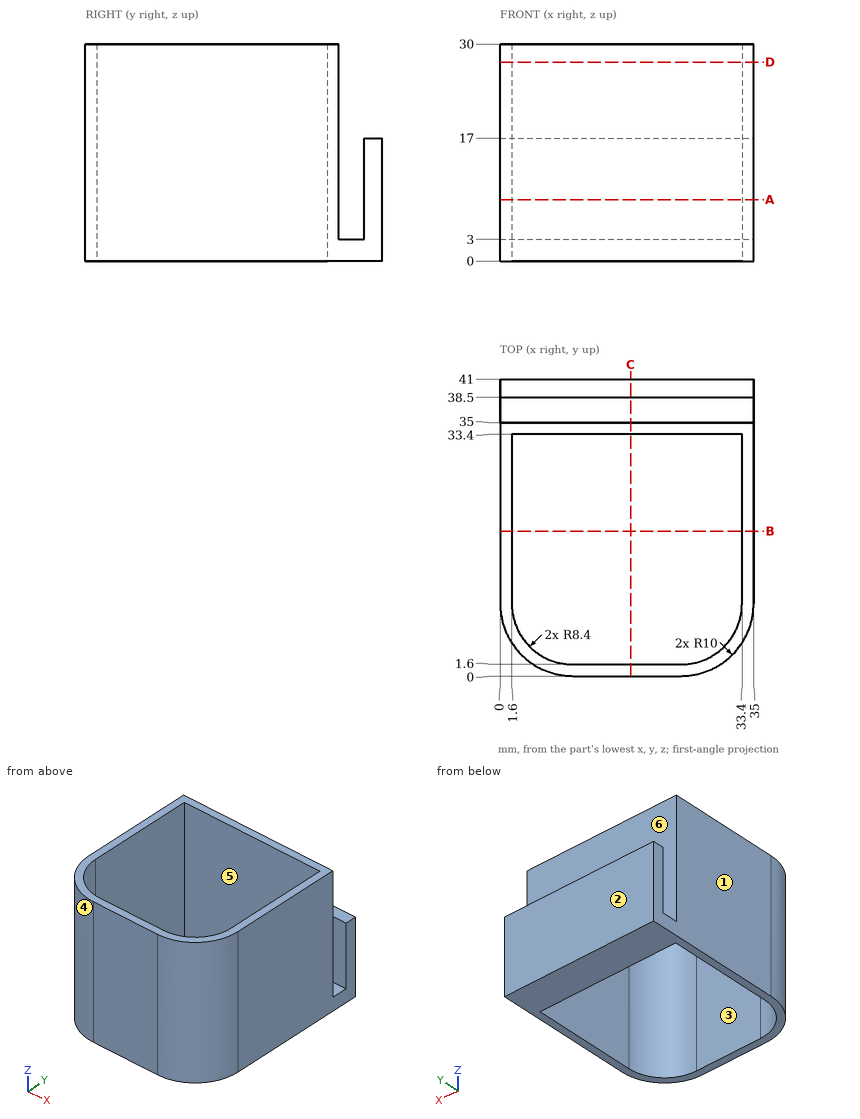
Verification items for this drawing (mm, ordinates from the low corner). A direction names the side the tool comes from. Coordinates: 2 decimals unless noted, no trailing zeros. Order: outer loops, then holes, each group sorted by start corner. A loop starts at its lowest first (then second) coordinate and runs counter-clockwise, first axis right, second up. Notation, with made-up numbers: (31, 56) - (46, 56) arc R12 cw to (46, 64) - close; hole circle Ø3 at (-24, 19). An arc over 180 degrees is marked (long way). Answer as a JSON object with one key per item and string values. Group by question number.
Item 1: Depth check by flat-ended pin: pin 1 Ø1.2 at (x, y) = (15, 40) entering from +Z; pin 2 Ø10 at (x, y) = (11.5, 11.5) entering from +Z. Enter the tip coordinate at first touch or a pass-through.
Item 2: Draft check along X on the marked faces 1, 2 and 3. Enter one of: +X half, -X half, draft (parallel to the pull), parting line (faces both ways), or undercut.
Item 3: Sectioned sample at A-A, the plane z = 8.5. Record the cut outline in (x, y), and give its area (3 significant figures).
Item 4: Sectioned sample at B-B, the plane y = 20. Record the cut outline in (x, z), and give its area (3 significant figures).
Item 5: Scan lines: probe 1 along Y at (x, z) = (23, 8.5); probe 2 along X at (y, z) = (27.5, 1.75); probe 3 along Y at (x, z) = (28, 10.25). Record each from-to range of solid material in increasing order.
Item 6: Tool access check on the marked faces 4, 5 and 6. Record the directions out of +Z, -Z, +X, -X, +Y, -Y that give a thin tool (end or side, any length) a straight path to the whole face; none if there is none.
Item 7: Sectioned sample at D-D, the plane z = 27.5. Record the cut outline in (x, y), and give its area (3 significant figures).
Item 8: Sectioned sample at C-C, the plane x = 18. Record the cut outline in (y, z).
Resolved:
{
 "1": {"pin 1": "z = 17", "pin 2": "through"},
 "2": {"face 1": "-X half", "face 2": "draft", "face 3": "undercut"},
 "3": {"outline": "(0, 10) arc R10 ccw to (10, 0) - (25, 0) arc R10 ccw to (35, 10) - (35, 35) - (0, 35) - close; (0, 38.5) - (35, 38.5) - (35, 41) - (0, 41) - close; hole (1.6, 10) arc R8.4 ccw to (10, 1.6) - (25, 1.6) arc R8.4 ccw to (33.4, 10) - (33.4, 33.4) - (1.6, 33.4) - close", "area": "289 mm^2"},
 "4": {"outline": "(0, 0) - (1.6, 0) - (1.6, 30) - (0, 30) - close; (33.4, 0) - (35, 0) - (35, 30) - (33.4, 30) - close", "area": "96.0 mm^2"},
 "5": {"probe 1": "0 to 1.6, 33.4 to 35, 38.5 to 41", "probe 2": "0 to 1.6, 33.4 to 35", "probe 3": "0.46 to 2.15, 33.4 to 35, 38.5 to 41"},
 "6": {"face 4": "+Z, -Z, -X, -Y", "face 5": "+Z, -Z", "face 6": "+Z, +X, -X"},
 "7": {"outline": "(0, 10) arc R10 ccw to (10, 0) - (25, 0) arc R10 ccw to (35, 10) - (35, 35) - (0, 35) - close; hole (1.6, 10) arc R8.4 ccw to (10, 1.6) - (25, 1.6) arc R8.4 ccw to (33.4, 10) - (33.4, 33.4) - (1.6, 33.4) - close", "area": "201 mm^2"},
 "8": {"outline": "(0, 0) - (1.6, 0) - (1.6, 30) - (0, 30) - close; (33.4, 0) - (41, 0) - (41, 17) - (38.5, 17) - (38.5, 3) - (35, 3) - (35, 30) - (33.4, 30) - close"}
}
